Answer from the drawing. Dimensions are ordinates in mm from the lowest x, y and z of the part. Give positions to 0.01 mm unless a question says otherwise; leave off trailing zeros. Loops run counter-clockwise (first coordinate to the right, second up) from the corner with the lowest first, then second, coordinate; pieces in that order, holes last.
Item 1: Consider line 1 along X through (y, z) = (0.8, 11.5); line 2 along Z through (x, y) = (13, 0.6) (3 decimals); line 3 along X through (y, z) = (2.25, 10). Determine where each line is inside the solid, lowest interval first.
Item 2: Section C-C, the plane y = 6.5 is taken. Give the vertices of the cut face in (x, z).
Item 3: Section D-D, the plane x = 4 is taken. Give the vertices of the cut face in (y, z) (3 decimals).
Item 4: Section A-A, the plane x = 47 is taken. Give the vertices of the cut face in (y, z) (3 decimals), and give its area (3 significant figures).
Item 5: Each of these flat-tipped pins is pushed along its axis until it touches: pin 1 Ø1.5 at (x, y) = (44, 2.5) entering from +Z; pin 2 Ø3 at (y, z) = (4.5, 27.5) entering from -X; pin 3 Ø1.1 at (x, y) = (50, 0.5) entering from +Z (3 decimals); pin 4 Ø3 at (x, z) = (34, 29.5) entering from -Y. Where does it stop, or does it pass through?
Item 6: The mould has two halves that part along Z. Classify the marked faces 1, 2 and 3: pulls with the +Z half, pulls with the -Z half, needs draft (parallel to the pull), parting line crosses it, or undercut.
Item 7: Section B-B, the plane z = 11.5 is taken. Give the vertices of the cut face in (x, y).
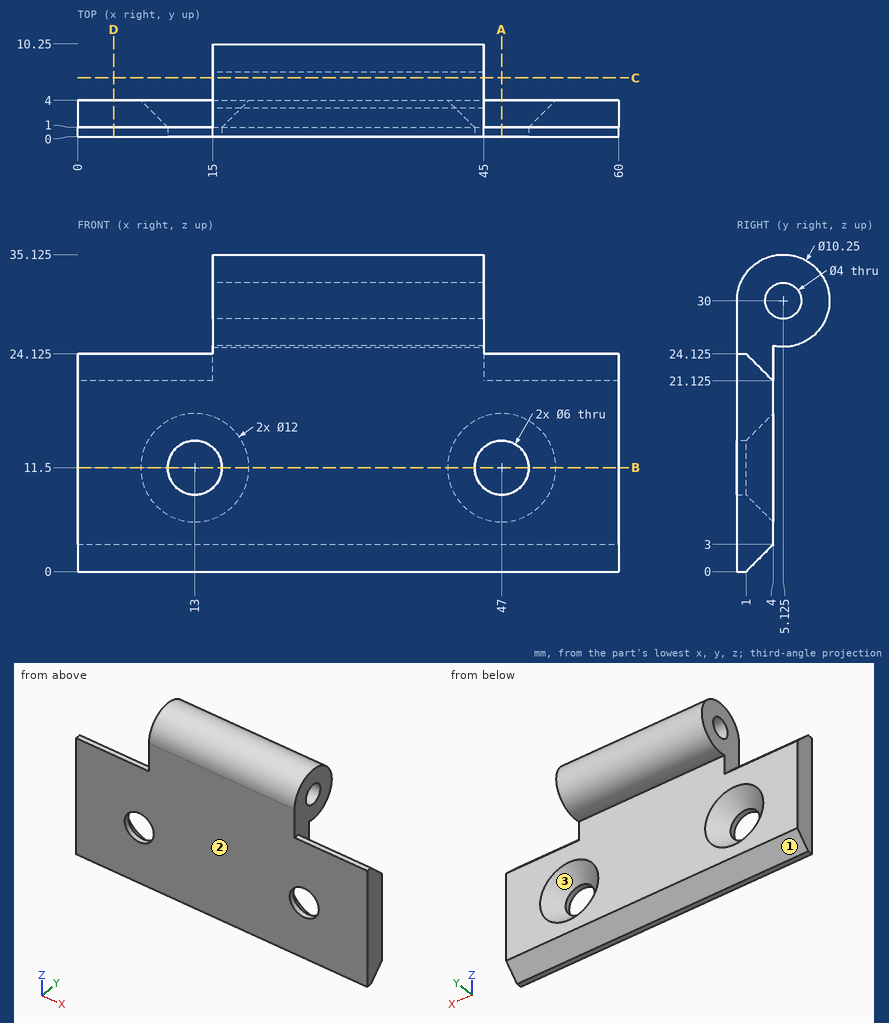
Worked answers:
1. line 1: x = 0 to 10, 16 to 44, 50 to 60
1. line 2: z = 0 to 8.5, 14.5 to 24.125
1. line 3: x = 0 to 9.02, 16.98 to 43.02, 50.98 to 60
2. outline: (15, 25.06) - (45, 25.06) - (45, 28.55) - (15, 28.55) - close; (15, 31.45) - (45, 31.45) - (45, 34.94) - (15, 34.94) - close
3. outline: (0, 0) - (1, 0) - (4, 3) - (4, 21.125) - (1, 24.125) - (0, 24.125) - close
4. outline: (0, 0) - (1, 0) - (4, 3) - (4, 5.5) - (1, 8.5) - (0, 8.5) - close; (0, 14.5) - (1, 14.5) - (4, 17.5) - (4, 21.125) - (1, 24.125) - (0, 24.125) - close
4. area: 54.5 mm2
5. pin 1: stops at z = 34.77
5. pin 2: stops at x = 15
5. pin 3: stops at z = 24.125
5. pin 4: stops at y = 0
6. face 1: pulls with the -Z half
6. face 2: needs draft
6. face 3: undercut
7. outline: (0, 0) - (10, 0) - (10, 1) - (7, 4) - (0, 4) - close; (16, 0) - (44, 0) - (44, 1) - (41, 4) - (19, 4) - (16, 1) - close; (50, 0) - (60, 0) - (60, 4) - (53, 4) - (50, 1) - close
